from build123d import *

# Parameters (mm, degrees)
F0_W     = 65
F0_H     = 40
F1_DEPTH = 26
F2_R     = 3
F3_DEPTH = 15
F4_R     = 3
F5_DEPTH = 15


with BuildPart() as f1:
    # F0 (on Top) → F1 (new body)
    with BuildSketch(Plane.XY):
        Rectangle(F0_W, F0_H)
    extrude(amount=F1_DEPTH)

    # F2 (on face) → F3 (join)
    with BuildSketch(Plane.YZ.offset(32.5)):
        with Locations((0, 16)):
            Circle(F2_R)
        with Locations((-15, 16)):
            Circle(F2_R)
        with Locations((15, 16)):
            Circle(F2_R)
    extrude(amount=F3_DEPTH)

    # F4 (on face) → F5 (join)
    with BuildSketch(Plane(origin=(-32.5, 0, 0), x_dir=(0, -1, 0), z_dir=(-1, 0, 0))):
        with Locations((15, 16)):
            Circle(F4_R)
        with Locations((-15, 16)):
            Circle(F4_R)
    extrude(amount=F5_DEPTH)


solid = f1.part
Source: CAD feature listing. Evaluate the final solid. Frame: model axes, mm. A direction names the side the tool comes from. Round coordinates to 2 decimals unless told otherwise and drop trailing zeros. Order: outer loops, then holes, each group sorted by start corner. A loop starts at its lowest first (then second) coordinate and runs counter-clockwise, first axis right, second up. Notation, with made-up numbers: (-39.75, -11) -> (-34.75, -11) arc R21 cw to (-34.75, 15) -> close; hole circle Ø4 at (-34, 74.5). An arc over 180 degrees is marked (long way). Answer as CSV lines item,"result".
Item 1: Section A-A, the plane y = 0. Return loops of the section in (x, z).
A:
outline,"(-32.5, 0) -> (32.5, 0) -> (32.5, 13) -> (47.5, 13) -> (47.5, 19) -> (32.5, 19) -> (32.5, 26) -> (-32.5, 26) -> close"
Item 2: Section B-B, the plane z = 16. Return loops of the section in (x, y), plus the area to 3 significant figures.
A:
outline,"(-47.5, -18) -> (-32.5, -18) -> (-32.5, -20) -> (32.5, -20) -> (32.5, -18) -> (47.5, -18) -> (47.5, -12) -> (32.5, -12) -> (32.5, -3) -> (47.5, -3) -> (47.5, 3) -> (32.5, 3) -> (32.5, 12) -> (47.5, 12) -> (47.5, 18) -> (32.5, 18) -> (32.5, 20) -> (-32.5, 20) -> (-32.5, 18) -> (-47.5, 18) -> (-47.5, 12) -> (-32.5, 12) -> (-32.5, -12) -> (-47.5, -12) -> close"
area,"3,050 mm²"
Item 3: Section D-D, the plane y = 15. Return loops of the section in (x, z), plus the area to 3 significant figures.
A:
outline,"(-47.5, 13) -> (-32.5, 13) -> (-32.5, 0) -> (32.5, 0) -> (32.5, 13) -> (47.5, 13) -> (47.5, 19) -> (32.5, 19) -> (32.5, 26) -> (-32.5, 26) -> (-32.5, 19) -> (-47.5, 19) -> close"
area,"1,870 mm²"
Item 4: Reachability of faces 4 (the face through (39.89, -0.65, 13.07)), 5 (the face through (-39.9, 17.4, 14.2)), 6 (the face through (0, 20, 13)) from +Z, -Z, +X, -X, +Y, -Y: full face, straight path, thin tool, end or side. Return the list, or none.
A:
face 4,"+X"
face 5,"-X"
face 6,"+Z, -Z, +X, -X, +Y"
Item 5: Pin query (flat end, axial travel): pin 1 Ø1 at (x, y) = (31.5, 1) entering from -Z; pin 2 Ø4 at (y, z) = (1.5, 21.5) entering from +X; pin 3 Ø2 at (y, z) = (15.5, 23.5) entering from -X. Return the tip coordinate at first contact, or that it passes through.
A:
pin 1,"z = 0"
pin 2,"x = 32.5"
pin 3,"x = -32.5"
Item 6: Line query: L1, parallel to X at y = -10, z = 15.5; L2, parallel to Y at x = -40.5, z = 14.75. Output: solid intervals per line, ascending.
A:
L1,"-32.5 to 32.5"
L2,"-17.73 to -12.27, 12.27 to 17.73"
Item 7: Pull-direction query (Y, two-part tool) for faces 1 (the face through (0, -20, 13)), 2 (the face through (-47.5, 15, 16)), 3 (the face through (32.5, -0.3, 12.8)); classes: pulls with the +Y half, pulls with the -Y half, needs draft (parallel to the pull), parting line crosses it, or undercut.
A:
face 1,"pulls with the -Y half"
face 2,"needs draft"
face 3,"undercut"
Item 8: Section C-C, the plane x = 40. Return loops of the section in (y, z).
A:
outline,"circle Ø6 at (-15, 16); circle Ø6 at (0, 16); circle Ø6 at (15, 16)"
